Design review of the part built by this model. Coordinates are the model's own, in mm. A direction names the side the tool comes from. Give positions to 0.01 mm unless a question says otherwise; leave off trailing zeros. Loops run counter-clockwise (first coordinate to the right, second up) from the corner with the lowest first, then second, coordinate; pieces in that order, holes last.
from build123d import *

# Parameters (mm, degrees)
F0_W     = 200
F0_H     = 160
F1_DEPTH = 35
F3_DEPTH = 50
F4_SIZE  = 5
F5_R     = 10
F6_DEPTH = 15
F7_R     = 6.5
F8_DEPTH = 20


with BuildPart() as f1:
    # F0 (on Top) → F1 (new body)
    with BuildSketch(Plane.XY):
        Rectangle(F0_W, F0_H)
    extrude(amount=F1_DEPTH)

    # F2 (on face) → F3 (join)
    with BuildSketch(Plane.XY.offset(35)):
        with BuildLine():
            Line((-45, 20), (-83.5, 20))
            ThreePointArc((-83.5, 20), (-83.499199, 19.634294), (-83.496797, 19.268595))
            ThreePointArc((-83.496797, 19.268595), (-84.615489, 14.584353), (-87.793986, 10.966239))
            ThreePointArc((-87.793986, 10.966239), (-92.260652, -0.450479), (-83.388126, -8.910435))
            ThreePointArc((-83.388126, -8.910435), (-78.978477, -10.846561), (-75.985202, -14.619346))
            ThreePointArc((-75.985202, -14.619346), (-72.131939, -22.062255), (-67.551957, -29.081393))
            ThreePointArc((-67.551957, -29.081393), (-65.742607, -33.544559), (-66.229285, -38.335879))
            ThreePointArc((-66.229285, -38.335879), (-61.795593, -51.32092), (-48.150249, -49.880952))
            ThreePointArc((-48.150249, -49.880952), (-44.922849, -47.748231), (-41.127489, -47))
            Line((-41.127489, -47), (41.127489, -47))
            ThreePointArc((41.127489, -47), (44.922849, -47.748231), (48.150249, -49.880952))
            ThreePointArc((48.150249, -49.880952), (61.795593, -51.32092), (66.229285, -38.335879))
            ThreePointArc((66.229285, -38.335879), (65.742607, -33.544559), (67.551957, -29.081393))
            ThreePointArc((67.551957, -29.081393), (72.131939, -22.062255), (75.985202, -14.619346))
            ThreePointArc((75.985202, -14.619346), (78.978477, -10.846561), (83.388126, -8.910435))
            ThreePointArc((83.388126, -8.910435), (92.260652, -0.450479), (87.793986, 10.966239))
            ThreePointArc((87.793986, 10.966239), (84.615489, 14.584353), (83.496797, 19.268595))
            ThreePointArc((83.496797, 19.268595), (83.499199, 19.634294), (83.5, 20))
            Line((83.5, 20), (45, 20))
            ThreePointArc((45, 20), (44.732617, 15.101734), (43.933644, 10.261677))
            ThreePointArc((43.933644, 10.261677), (38.8735, -2.668281), (30.112429, -13.44012))
            ThreePointArc((30.112429, -13.44012), (0, -25), (-30.112429, -13.44012))
            ThreePointArc((-30.112429, -13.44012), (-38.8735, -2.668281), (-43.933644, 10.261677))
            ThreePointArc((-43.933644, 10.261677), (-44.732617, 15.101734), (-45, 20))
        make_face()
        with BuildLine():
            ThreePointArc((-84.67549, 44.888838), (-82.209915, 40.751866), (-81.963998, 35.942175))
            ThreePointArc((-81.963998, 35.942175), (-83.115113, 28.008), (-83.5, 20))
            Line((-83.5, 20), (-45, 20))
            Line((-45, 20), (-45, 39.104097))
            Line((-45, 39.104097), (-45, 46.58))
            Line((-45, 46.58), (-71.264379, 62.100147))
            ThreePointArc((-71.264379, 62.100147), (-85.537354, 59.391052), (-84.67549, 44.888838))
        make_face()
        with BuildLine():
            Line((45, 39.104097), (45, 20))
            Line((45, 20), (83.5, 20))
            ThreePointArc((83.5, 20), (83.115113, 28.008), (81.963998, 35.942175))
            ThreePointArc((81.963998, 35.942175), (82.209915, 40.751866), (84.67549, 44.888838))
            ThreePointArc((84.67549, 44.888838), (85.537354, 59.391052), (71.264379, 62.100147))
            Line((71.264379, 62.100147), (45, 46.58))
            Line((45, 46.58), (45, 39.104097))
        make_face()
        with BuildLine():
            Line((67.673667, 46.58), (62.609608, 46.58))
            Line((62.609608, 46.58), (66.735146, 48.331437))
            ThreePointArc((66.735146, 48.331437), (67.164778, 47.434483), (67.673667, 46.58))
        make_face(mode=Mode.SUBTRACT)
        with BuildLine():
            Line((66.735146, 48.331437), (62.609608, 46.58))
            Line((62.609608, 46.58), (67.673667, 46.58))
            ThreePointArc((67.673667, 46.58), (67.164778, 47.434483), (66.735146, 48.331437))
        make_face()
    extrude(amount=F3_DEPTH)

    # F4
    f4_edges = [f1.edges().sort_by_distance(p)[0] for p in [
        (100, -80, 17.5),
        (100, 80, 17.5),
        (-100, 80, 17.5),
        (-100, -80, 17.5),
    ]]
    chamfer(f4_edges, length=F4_SIZE)

    # F5 (on face) → F6 (cut)
    with BuildSketch(Plane.XY.offset(35)):
        with Locations((-80, -60)):
            Circle(F5_R)
        with Locations((80, -60)):
            Circle(F5_R)
        with Locations((-30, 60)):
            Circle(F5_R)
        with Locations((30, 60)):
            Circle(F5_R)
    extrude(amount=-F6_DEPTH, mode=Mode.SUBTRACT)

    # F7 (on face) → F8 (cut)
    with BuildSketch(Plane.XY.offset(20)):
        with Locations((-30, 60)):
            Circle(F7_R)
        with Locations((30, 60)):
            Circle(F7_R)
        with Locations((-80, -60)):
            Circle(F7_R)
        with Locations((80, -60)):
            Circle(F7_R)
    extrude(amount=-F8_DEPTH, mode=Mode.SUBTRACT)


solid = f1.part
Q1. Take a section at C-C (x = -13.5). Give the boundary of the cut face in (y, z).
Results:
outline: (-80, 0) - (80, 0) - (80, 35) - (-22.93, 35) - (-22.93, 85) - (-47, 85) - (-47, 35) - (-80, 35) - close
Q2. Tool access review of faces 1 (the face through (45, 33, 60)), 2 (the face through (-80, -67, 20)), 3 (the face through (-83.104, 28.12, 59.65)), 4 (the face through (-1, -47, 60)): name each direction out of +Z, -Z, +X, -X, +Y, -Y from which nothing blocks a thin tool from reaching the whole face with its end or side.
Results:
face 1: +Z, +Y
face 2: +Z
face 3: +Z, -X
face 4: +Z, -Y
Q3. Draft analysis for pull direction Y (two halves, no side actions). For faces 5 (the face through (-100, -1, 17)), 6 (the face through (30, 53, 20)), 7 (the face through (83.126, 27.896, 59.65)), 8 (the face through (-44.725, 15.033, 59.65)), state which applies: pulls with the +Y half, pulls with the -Y half, needs draft (parallel to the pull), parting line crosses it, or undercut.
Results:
face 5: needs draft
face 6: undercut
face 7: undercut
face 8: pulls with the +Y half
Q4. Insertion check: pin 1 (5 mm diameter, centred on y = -39, z = 54.5, fed in from +X); pin 2 (15 mm diameter, centred on x = 16.5, z = 61, fed in from -Y); pin 3 (10 mm diameter, centred on x = 77.5, y = -62, fed in from +Z); pin 4 (11.5 mm diameter, centred on x = -30, y = 60, fed in from -Z). Each pin has a flat end and moves straight along its axis. Give the tip position at first contact, or say it passes through.
Results:
pin 1: stops at x = 66.86
pin 2: stops at y = -47
pin 3: stops at z = 20
pin 4: passes through
Q5. Take a section at B-B (z = 31.5). Give the boundary of the cut face in (x, y), plus the area to 3 significant figures.
Results:
outline: (-100, -75) - (-95, -80) - (95, -80) - (100, -75) - (100, 75) - (95, 80) - (-95, 80) - (-100, 75) - close; hole circle Ø20 at (-80, -60); hole circle Ø20 at (-30, 60); hole circle Ø20 at (30, 60); hole circle Ø20 at (80, -60)
area: 30,700 mm2
Q6. Take a section at A-A (y = -60). Give the boundary of the cut face in (x, z), plus the area to 3 significant figures.
Results:
outline: (-100, 0) - (-86.5, 0) - (-86.5, 20) - (-90, 20) - (-90, 35) - (-100, 35) - close; (-73.5, 0) - (73.5, 0) - (73.5, 20) - (70, 20) - (70, 35) - (-70, 35) - (-70, 20) - (-73.5, 20) - close; (86.5, 0) - (100, 0) - (100, 35) - (90, 35) - (90, 20) - (86.5, 20) - close
area: 5,880 mm2
Q7. Wall thickness on line 1 (Y direction, x = 30, z = 28); line 2 (Y direction, x = 80, z = 8); line 3 (Z direction, x = -31, y = 35): over which ranges is each line inside the solid? List them lowest first.
Results:
line 1: y = -80 to 50, 70 to 80
line 2: y = -80 to -66.5, -53.5 to 80
line 3: z = 0 to 35
